from build123d import *
from build123d.topology import SkipClean

# Parameters (mm, degrees)
SKETCH2_W               = 140
SKETCH2_H               = 89
SKETCH2_W_2             = 55
SKETCH2_H_2             = 69
BOSS_EXTRUDE2_DEPTH     = 50
CUT_EXTRUDE1_DEPTH      = 124.778027129
CUT_EXTRUDE1_DEPTH_BACK = 124.778027129
SKETCH3_R               = 5
SKETCH4_R               = 8
CUT_EXTRUDE2_DEPTH      = 15
SKETCH5_W               = 10
SKETCH5_H               = 89
BOSS_EXTRUDE4_DEPTH     = 30
SKETCH4_5_R             = 8
CUT_EXTRUDE5_DEPTH      = 30
MIRROR5_START           = 60
MIRROR5_DEPTH           = 10


# Read off the part's stored shape, not the designer's step: Mirror5
with BuildPart() as part:
    # Sketch2 → Boss-Extrude2 (new body)
    with BuildSketch(Plane.XY):
        with Locations((0, -0.480959067)):
            Rectangle(SKETCH2_W, SKETCH2_H)
        with Locations((32.5, -0.480959067)):
            Rectangle(SKETCH2_W_2, SKETCH2_H_2, mode=Mode.SUBTRACT)
        with Locations((-32.5, -0.480959067)):
            Rectangle(SKETCH2_W_2, SKETCH2_H_2, mode=Mode.SUBTRACT)
    extrude(amount=BOSS_EXTRUDE2_DEPTH)

    # Sketch3 → Cut-Extrude1 (cut, two sides: drawn at the far end of the back side and taken through both)
    with BuildSketch(Plane.XZ.offset(44.980959067).offset(-CUT_EXTRUDE1_DEPTH_BACK)):
        with Locations(Location((-35, 22, 0), (0, 0, 270))):
            Circle(SKETCH3_R)
        with Locations(Location((35, 22, 0), (0, 0, 270))):
            Circle(SKETCH3_R)
    extrude(amount=CUT_EXTRUDE1_DEPTH + CUT_EXTRUDE1_DEPTH_BACK, mode=Mode.SUBTRACT)

    # Sketch4 → Cut-Extrude2 (cut)
    with BuildSketch(Plane.ZY.offset(70)):
        with Locations((50, 19.519040933)):
            Circle(SKETCH4_R)
        with Locations((50, -20.480959067)):
            Circle(SKETCH4_R)
    cut_extrude2 = extrude(amount=-CUT_EXTRUDE2_DEPTH, mode=Mode.SUBTRACT)

    # Mirror1: Cut-Extrude2 across plane
    add(cut_extrude2.mirror(Plane(origin=(0, 0, 0), x_dir=(0, 0, 1), z_dir=(1, 0, 0))), mode=Mode.SUBTRACT)

    # Sketch5 → Boss-Extrude4 (add)
    with BuildSketch(Plane.XY.offset(50)):
        with Locations((-65, -0.480959067)):
            Rectangle(SKETCH5_W, SKETCH5_H)
    extrude(amount=BOSS_EXTRUDE4_DEPTH)

    # Sketch4<5> → Cut-Extrude5 (cut)
    with BuildSketch(Plane.ZY.offset(70)):
        with Locations((50, 19.519040933)):
            Circle(SKETCH4_5_R)
        with Locations((50, -20.480959067)):
            Circle(SKETCH4_5_R)
    extrude(amount=-CUT_EXTRUDE5_DEPTH, mode=Mode.SUBTRACT)

    # Mirror5 outline → Mirror5 (add)
    with SkipClean():  # the faces are left unmerged after this step: merging them gives an invalid solid
        with BuildSketch(Plane.YZ.offset(MIRROR5_START)):
            with BuildLine():
                ThreePointArc((-28.480959067, 50), (-20.480959067, 58), (-12.480959067, 50))
                Line((-12.480959067, 50), (11.519040933, 50))
                ThreePointArc((11.519040933, 50), (19.519040933, 58), (27.519040933, 50))
                Line((27.519040933, 50), (44.019040933, 50))
                Line((44.019040933, 50), (44.019040933, 80))
                Line((44.019040933, 80), (-44.980959067, 80))
                Line((-44.980959067, 80), (-44.980959067, 50))
                Line((-44.980959067, 50), (-28.480959067, 50))
            make_face()
        extrude(amount=MIRROR5_DEPTH)
    add(part.part.scale(1), mode=Mode.REPLACE)  # the faces are merged on a copy


solid = part.part
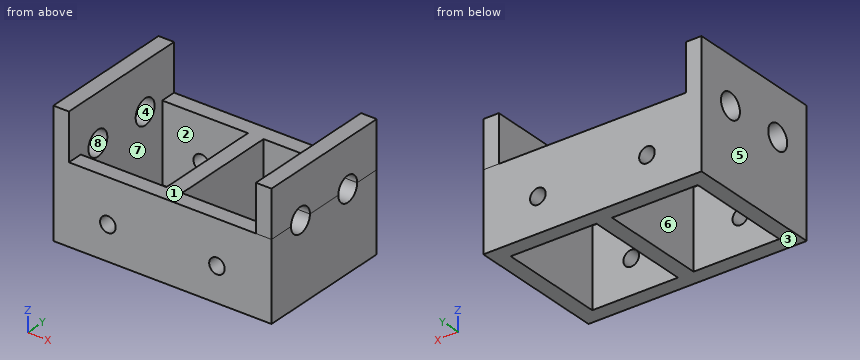
Read the model definition and answer for the solid it produces. Units are mm, in the model's axes. Face numbers are marked on the shaded views. A direction names the side the tool comes from. Round coordinates to 2 decimals unless told otherwise and drop trailing zeros. Loops run counter-clockwise (first coordinate to the right, second up) from the corner with the lowest first, then second, coordinate; pieces in that order, holes last.
Q1. Section D-D on z = 22 is taken. Write down the section's boundary in (x, y).
Q2. Section B-B on z = 38 is taken. Write down the section's boundary in (x, y).
Q3. Consider probe 1 along X at (y, z) = (-41, 22); probe 2 along X at (y, z) = (30.5, 24); probe 3 along Z at (x, y) = (35, 36.75). Determine where each line is inside the solid, lowest interval first.
Q4. Which of the six approach directions +Z, -Z, +X, -X, +Y, -Y give full straight-line access (tool end or side, diameter ignored) to the marked faces 1, 2, 3 and 4?
Q5. Each of these flat-tipped pins is pushed along its axis until it touches: pin 1 (3 mm diameter, centred on x = -5.5, y = 21, fed in from +Z); pin 2 (8 mm diameter, centred on x = 35, z = 22, fed in from +Y); pin 3 (13 mm diameter, centred on y = 19.52, z = 50, fed in from -X). Where does it stop, or does it pass through?
Q6. Determine the mould class of the marked faces 5, 6, 7 and 8 for opening direction X: released by +X, released by -X, zero draft, split by the parting line, or undercut.
Q7. Section A-A on x = 35 is taken. Write down the section's boundary in (y, z).
Q8. Section C-C on x = 10.5 is taken. Write down the section's boundary in (y, z).
Output:
1. outline: (-70, -44.98) - (-40, -44.98) - (-40, -34.98) - (-60, -34.98) - (-60, 34.02) - (-40, 34.02) - (-40, 44.02) - (-70, 44.02) - close; (-30, -44.98) - (30, -44.98) - (30, -34.98) - (5, -34.98) - (5, 34.02) - (30, 34.02) - (30, 44.02) - (-30, 44.02) - (-30, 34.02) - (-5, 34.02) - (-5, -34.98) - (-30, -34.98) - close; (40, -44.98) - (70, -44.98) - (70, 44.02) - (40, 44.02) - (40, 34.02) - (60, 34.02) - (60, -34.98) - (40, -34.98) - close
2. outline: (-70, -44.98) - (70, -44.98) - (70, 44.02) - (-70, 44.02) - close; hole (-60, -34.98) - (-5, -34.98) - (-5, 34.02) - (-60, 34.02) - close; hole (5, -34.98) - (60, -34.98) - (60, 34.02) - (5, 34.02) - close
3. probe 1: x = -70 to -40, -30 to 30, 40 to 70
3. probe 2: x = -70 to -60, -5 to 5, 60 to 70
3. probe 3: z = 0 to 17, 27 to 50
4. face 1: +Z, +Y, -Y
4. face 2: +Z, -Z
4. face 3: -Z, +X, -X, +Y, -Y
4. face 4: -X
5. pin 1: stops at z = 50
5. pin 2: passes through
5. pin 3: stops at x = -5
6. face 5: released by -X
6. face 6: undercut
6. face 7: undercut
6. face 8: zero draft
7. outline: (-44.98, 0) - (-34.98, 0) - (-34.98, 17) - (-44.98, 17) - close; (-44.98, 27) - (-34.98, 27) - (-34.98, 50) - (-44.98, 50) - close; (34.02, 0) - (44.02, 0) - (44.02, 17) - (34.02, 17) - close; (34.02, 27) - (44.02, 27) - (44.02, 50) - (34.02, 50) - close
8. outline: (-44.98, 0) - (-34.98, 0) - (-34.98, 50) - (-44.98, 50) - close; (34.02, 0) - (44.02, 0) - (44.02, 50) - (34.02, 50) - close
